Geometry: final body of the model. Coordinates: model frame, mm. A direction names the side the tool comes from. Coordinates: 2 decimals unless noted, no trailing zeros. Order: outer loops, then holes, each group sorted by start corner. A loop starts at its lowest first (then second) coordinate and runs counter-clockwise, first axis right, second up. Notation, with made-up numbers: (23, -0.75) -> (40, -0.75) arc R26 cw to (40, 20.25) -> close; hole circle Ø4 at (-39, -19). An arc over 180 degrees is marked (long way). Use one line per item in the form item = value.
```python
from build123d import *


with BuildPart() as part:
    # Sketch1 → Revolve1 (revolve)
    with BuildSketch(Plane(origin=(0, 0, 0), x_dir=(0, 0, -1), z_dir=(1, 0, 0))):
        with BuildLine():
            Line((0, 2.9337), (11.73, 2.9337))
            Line((11.73, 2.9337), (11.73, 7.9375))
            Line((11.73, 7.9375), (9.19, 7.9375))
            Line((9.19, 7.9375), (9.19, 5.561))
            ThreePointArc((9.19, 5.561), (9.160710678, 5.490289322), (9.09, 5.461))
            Line((9.09, 5.461), (3.79, 5.461))
            Line((3.79, 5.461), (3.79, 5))
            Line((3.79, 5), (2.54, 5))
            Line((2.54, 5), (2.54, 5.461))
            Line((2.54, 5.461), (0, 5.461))
            Line((0, 5.461), (0, 2.9337))
        make_face()
    revolve(axis=Axis((0, 0, 0), (0, 0, -1)))


solid = part.part
```
1) Pull-direction query (Z, two-part tool) for faces 1 (the cylindrical face through (-4.88, -1.08, -3.16)), 2 (the cylindrical face through (1.64, 5.21, -6.4)), 3 (the flat face through (0.1, -3.4, -11.73)), 4 (the flat face through (-2.4, 2.4, 0)); classes: released by +Z, released by -Z, zero draft, split by the parting line, or undercut.
Results found:
face_1 = undercut
face_2 = zero draft
face_3 = released by -Z
face_4 = released by +Z
2) Contact query for flat-ended pins moving along their axis: P1, Ø6, axis at y = -2, z = -6.5, coming from the -X side; P2, Ø2, axis at x = 1, z = -3, coming from the -Y side; P3, Ø1.5, axis at x = -2.5, z = -7.5, coming from the +Y side; P4, Ø3.5, axis at x = 0, y = 0, coming from the +Z side. Output: stop coordinate, or through.
Results found:
P1 = -7.91
P2 = -5.46
P3 = 5.17
P4 = through
3) Section C-C, the plane z = -1. Output: boundary loops of the cut face in (x, y), and give its area (3 significant figures).
Results found:
outline = circle Ø10.92 at (0, 0); hole circle Ø5.87 at (0, 0)
area = 66.7 mm2
4) Section D-D, the plane z = -3.25. Output: boundary loops of the cut face in (x, y).
Results found:
outline = circle Ø10 at (0, 0); hole circle Ø5.87 at (0, 0)
5) Access query for faces 5 (the flat face through (5.4, -1.9, -9.19)), 6 (the cylindrical face through (-2.864, -0.636, -5.947)). Directions: +Z, -Z, +X, -X, +Y, -Y. A direction counts if a zero-diameter tool reaches every point of the face in a straight line with its end or side. Return the directions, or none.
Results found:
face_5 = +Z
face_6 = +Z, -Z
6) Material intervals for probe 1 along X at (y, z) = (0, -2.75); probe 2 along X at (y, z) = (0, -6.75); probe 3 along Z at (x, y) = (6.25, -2.25), sorted ascending. Write a range as from..to.
Results found:
probe_1 = -5..-2.93, 2.93..5
probe_2 = -5.46..-2.93, 2.93..5.46
probe_3 = -11.73..-9.19
7) Section A-A, the plane y = 0. Output: boundary loops of the cut face in (x, z), and give its area (3 significant figures).
Results found:
outline = (-7.94, -11.73) -> (-2.93, -11.73) -> (-2.93, 0) -> (-5.46, 0) -> (-5.46, -2.54) -> (-5, -2.54) -> (-5, -3.79) -> (-5.46, -3.79) -> (-5.46, -9.09) arc R0.1 cw to (-5.56, -9.19) -> (-7.94, -9.19) -> close; (2.93, -11.73) -> (7.94, -11.73) -> (7.94, -9.19) -> (5.56, -9.19) arc R0.1 cw to (5.46, -9.09) -> (5.46, -3.79) -> (5, -3.79) -> (5, -2.54) -> (5.46, -2.54) -> (5.46, 0) -> (2.93, 0) -> close
area = 70.7 mm2
